Solid Edge part; units mm, degrees
sketch "Sketch1" plane through (0, 0, 0) normal (0, -1, 0) x (1, 0, 0)
  line L0 (1.25, 1.63) -> (1.25, 0.95)
  line L1 (1.25, 0.95) -> (8.25, 0.95)
  line L2 (8.25, 0) -> (8.25, 0.95)
  spline S0 degree 3 poles (0, 0) (0, 0.7831) (0.4356, 1.448) (1.25, 1.63) knots 0 0 0 0 1 1 1 1
revolve "RevolvedProtrusion1" add sketch "Sketch1" angle 360 about axis through (0, 0, 0) along (1, 0, 0)
sketch "Sketch2" plane through (0, 0, 0) normal (1, 0, 0) x (0, 0, 1)
  line L0 (-0.375, 1.9976) -> (0.375, 1.9976)
  line L1 (0.375, 1.9976) -> (0.375, 0.6495)
  arc A0 (0.375, 0.6495) -> (0.375, -0.6495) centre (0, 0) cw
  line L2 (0.375, -0.6495) -> (0.375, -1.9976)
  line L3 (0.375, -1.9976) -> (-0.375, -1.9976)
  line L4 (-0.375, -1.9976) -> (-0.375, -0.6495)
  line L5 (-0.375, 0.6495) -> (-0.375, 1.9976)
  arc A1 (-0.375, -0.6495) -> (-0.375, 0.6495) centre (0, 0) cw
extrude "Cutout1" cut sketch "Sketch2" along normal blind 0.6
fillet "Round_1" radius 0.15 2 edges at (1.25, 0, -1.63) (8.25, 0, -0.95)
properties material "Galvanized steel"
Geometry: final body of the model. Coordinates: model frame, mm. Round coordinates to 2 decimals unless told otherwise and drop trailing zeros. Loops run counter-clockwise (first coordinate to the right, second up) from the corner with the lowest first, then second, coordinate; pieces in that order, holes last. Notation, with made-up numbers: (73, 10) -> (116, 10) arc R32 cw to (116, 46) -> close; hole circle Ø3 at (85, 52.25). An arc over 180 degrees is marked (long way). Write each question's results on one line, items separated by ' | '.
Item 1: Pin query (flat end, axial travel): pin 1 Ø0.5 at (x, y) = (0.5, 1) entering from +Z; pin 2 Ø1 at (x, z) = (4.5, -1) entering from -Y; pin 3 Ø0.5 at (x, y) = (0.5, 1) entering from -Z. Return the tip coordinate at first contact, or that it passes through.
Answers below:
pin 1: stops at z = 1.12 | pin 2: stops at y = -0.81 | pin 3: stops at z = -1.12
Item 2: Pull-direction query (Y, two-part tool) for faces 1 (the face through (4.72, -0.04, -0.95)), 2 (the face through (8.25, 0, 0)), 3 (the face through (0.6, 0, 0)); classes: pulls with the +Y half, pulls with the -Y half, needs draft (parallel to the pull), parting line crosses it, or undercut.
Answers below:
face 1: parting line crosses it | face 2: needs draft | face 3: undercut
Item 3: Cut plane A-A on x = 7.5. Return the cut outline in (y, z).
Answers below:
outline: circle Ø1.9 at (0, 0)
Item 4: Line query: probe 1 along Y at (x, z) = (3, 0); probe 2 along X at (y, z) = (0.7, 1.25); probe 3 along X at (y, z) = (0.5, 0.5). Output: solid intervals per line, ascending. Write a range as [from, to].
Answers below:
probe 1: y = [-0.95, 0.95] | probe 2: x = [0.75, 1.25] | probe 3: x = [0.6, 8.25]
